from build123d import *

# Parameters (mm, degrees)
CHAMFER_ANGLE   = 15
CHAMFER_SIZE    = 3
CHAMFER001_SIZE = 0.5


with BuildPart() as part:
    # Sketch010 → Revolution (revolve)
    with BuildSketch(Plane.YZ):
        Polygon((18.25, -70), (20.05, -70), (20.05, 0), (15, 8.746857), (15, 38.746857), (11.7, 38.746857), (11.7, 8.746857), (16.75, 0), align=None)
    revolve(axis=Axis((0, 0, 0), (0, 0, 1)))

    # Chamfer
    chamfer_edges = [part.edges().sort_by_distance(p)[0] for p in [
        (0, -15, 38.746857),
    ]]
    chamfer_side = part.faces().sort_by_distance((0, -15, 23.746857))[0]
    chamfer(chamfer_edges, length=CHAMFER_SIZE, angle=CHAMFER_ANGLE, reference=chamfer_side)

    # Chamfer001
    chamfer001_edges = [part.edges().sort_by_distance(p)[0] for p in [
        (0, -18.25, -70),
        (0, -20.05, -70),
    ]]
    chamfer(chamfer001_edges, length=CHAMFER001_SIZE)


with BuildPart() as part_1:
    # Body002 placement: moved
    add(part.part.moved(Location((0, 0, -35))))


solid = part_1.part
Build history of the part. All positions in model axes, mm. A direction names the side the tool comes from. Give positions to 0.01 mm unless a question says otherwise; leave off trailing zeros. Loops run counter-clockwise (first coordinate to the right, second up) from the corner with the lowest first, then second, coordinate; pieces in that order, holes last. Notation, with made-up numbers: (10, 40.5) -> (21, 40.5) arc R32 ccw to (21, 79.5) -> close; hole circle Ø9 at (8.25, 5.25). An arc over 180 degrees is marked (long way). Answer in a Markdown table with one row per item.
Item 1: Probe line 1 along X through (y, z) = (0, -10); line 2 along X through (y, z) = (-15, -99); line 3 along Y through (x, z) = (11, -98). List the from-to ranges inside material, lowest first. Write a range as [from, to].
Findings below:
| item | result |
|---|---|
| line 1 | x = [-15, -11.7], [11.7, 15] |
| line 2 | x = [-13.3, -10.17], [10.17, 13.3] |
| line 3 | y = [-16.76, -14.37], [14.37, 16.76] |
Item 2: Mould opens along X. For faces 1 (the conical face through (7.311, -9.535, -26.8)), 2 (the flat face through (-12, 2, 3.747)), 3 (the conical face through (9.276, -12.098, -26.678)) say: pulls with the +X half, pulls with the -X half, needs draft (parallel to the pull), parting line crosses it, or undercut.
Findings below:
| item | result |
|---|---|
| face 1 | undercut |
| face 2 | needs draft |
| face 3 | parting line crosses it |
Item 3: Tool access for faces 4 (the flat face through (19, -1, -105)), 5 (the conical face through (17.09, -3.79, -70.24)), 6 (the cylindrical face through (-0.66, -14.985, -12.564)): list every direction of +Z, -Z, +X, -X, +Y, -Y with a clear straight run to the whole face (end or side of a thin tool).
Findings below:
| item | result |
|---|---|
| face 4 | -Z, +X, -X, +Y, -Y |
| face 5 | -Z |
| face 6 | +Z |
Item 4: Slice it at D-D on z = -90.5. Write the cut outline in (x, y), plus the area to 3 significant figures.
Findings below:
| item | result |
|---|---|
| outline | circle Ø40.1 at (0, 0); hole circle Ø35.88 at (0, 0) |
| area | 252 mm² |
Item 5: Slice it at A-A on x = 0. Write the cut outline in (y, z).
Findings below:
| item | result |
|---|---|
| outline | (-20.05, -104.5) -> (-19.55, -105) -> (-18.75, -105) -> (-18.24, -104.5) -> (-16.75, -35) -> (-11.7, -26.25) -> (-11.7, 3.75) -> (-14.2, 3.75) -> (-15, 0.75) -> (-15, -26.25) -> (-20.05, -35) -> close; (11.7, -26.25) -> (16.75, -35) -> (18.24, -104.5) -> (18.75, -105) -> (19.55, -105) -> (20.05, -104.5) -> (20.05, -35) -> (15, -26.25) -> (15, 0.75) -> (14.2, 3.75) -> (11.7, 3.75) -> close |
Item 6: Slice it at C-C on z = -16.5. Write the cut outline in (x, y).
Findings below:
| item | result |
|---|---|
| outline | circle Ø30 at (0, 0); hole circle Ø23.4 at (0, 0) |
Item 7: Flat gauge pins, fed straight in: P1, Ø8, axis at x = 11.5, y = 1, coming from the -Z side; P2, Ø2, axis at x = -10.5, z = -83, coming from the -Y side; P3, Ø8, axis at y = -4.5, z = -15, coming from the +X side. Where does each tip first touch, or does it go through?
Findings below:
| item | result |
|---|---|
| P1 | stops at z = -32.91 |
| P2 | stops at y = -17.66 |
| P3 | stops at x = 14.99 |
